from build123d import *

# Parameters (mm, degrees)
PAD_DEPTH = 3
FILLET_R  = 1.25


with BuildPart() as part:
    # Sketch → Pad (new body)
    with BuildSketch(Plane.XY):
        with BuildLine():
            Line((0, 0), (0, 14))
            Line((0, 14), (40, 14))
            Line((40, 14), (40, 6))
            ThreePointArc((40, 6), (42, 4), (44, 6))
            Line((44, 6), (44, 13.953997))
            Line((44, 13.953997), (49, 13.953997))
            Line((49, 13.953997), (49, 6))
            ThreePointArc((42, -1), (46.949747, 1.050253), (49, 6))
            Line((16.769501, -1), (42, -1))
            ThreePointArc((16.769501, -1), (12.734056, -2.671536), (11.06252, -6.706981))
            Line((11.06252, -6.706981), (11.06252, -8))
            Line((5.5, -8), (11.06252, -8))
            Line((5.5, 8), (5.5, -8))
            Line((3, 8), (5.5, 8))
            Line((3, 0), (3, 8))
            Line((0, 0), (3, 0))
        make_face()
    extrude(amount=PAD_DEPTH)

    # Fillet
    fillet_edges = [part.edges().sort_by_distance(p)[0] for p in [
        (20, 14, 3),
        (20, 14, 0),
        (40, 14, 1.5),
        (40, 10, 0),
        (40, 10, 3),
        (42, 4, 0),
        (42, 4, 3),
        (44, 13.953997, 1.5),
        (44, 9.976998, 0),
        (44, 9.976998, 3),
        (49, 13.953997, 1.5),
        (46.5, 13.953997, 0),
        (46.5, 13.953997, 3),
        (49, 9.976998, 0),
        (49, 9.976998, 3),
        (46.949747, 1.050253, 0),
        (46.949747, 1.050253, 3),
        (29.38475, -1, 0),
        (29.38475, -1, 3),
        (12.734056, -2.671536, 0),
        (12.734056, -2.671536, 3),
        (11.06252, -8, 1.5),
        (11.06252, -7.353491, 0),
        (11.06252, -7.353491, 3),
    ]]
    fillet(fillet_edges, radius=FILLET_R)


solid = part.part
The model under review builds one solid part; all positions refer to its coordinate system, in mm. A direction names the side the tool comes from. Give positions to 0.01 mm unless a question says otherwise; leave off trailing zeros. Write each loop counter-clockwise with the first axis right and the second up, starting at its lowest first coordinate (ties: lowest second). Pieces come first, ordered by that corner, then holes.
1. Add section A-A, the plane y = 9. Write out the cut boundary in (x, z).
2. Wall thickness on L1, parallel to X at y = 9, z = 1.3; L2, parallel to X at y = 12, z = 2.5; L3, parallel to Y at x = 35.5, z = 1.5: over which ranges is each line inside the solid? List them lowest first.
3. For P1, Ø6, axis at x = 29.5, y = -3.5, coming from the -Z side; P2, Ø1.5, axis at x = 1.5, z = 1, coming from the -Y side; P3, Ø0.6, axis at x = 46.5, z = 1.5, coming from the +Y side, all flat-tipped, find the tip position at first contact; note any pin that passes through.
4. Tool access review of faces 1 (the cylindrical face through (10.541, -7.219, 2.766)), 2 (the cylindrical face through (39.624, 13.644, 1.504)), 3 (the cylindrical face through (44.356, 9.399, 0.376)): name each direction out of +Z, -Z, +X, -X, +Y, -Y from which nothing blocks a thin tool from reaching the whole face with its end or side.
5. Add section B-B, the plane z = 0.45. Write out the cut boundary in (x, y), plus the area to 3 significant figures.
6. Draft analysis for pull direction Y (two halves, no side actions). For faces 4 (the cylindrical face through (48.62, 13.6, 1.5)), 5 (the flat face through (19, 5, 0)), 6 (the cylindrical face through (29.208, -0.644, 0.376)), state which applies: +Y half, -Y half, draft (parallel to the pull), parting line (faces both ways), or undercut.
Worked answers:
1. outline: (0, 0) - (38.75, 0) arc R1.25 ccw to (40, 1.25) - (40, 1.75) arc R1.25 ccw to (38.75, 3) - (0, 3) - close; (44, 1.25) arc R1.25 ccw to (45.25, 0) - (47.75, 0) arc R1.25 ccw to (49, 1.25) - (49, 1.75) arc R1.25 ccw to (47.75, 3) - (45.25, 3) arc R1.25 ccw to (44, 1.75) - close
2. L1: x = 0 to 40, 44 to 49
2. L2: x = 0 to 39.75, 44.25 to 48.75
2. L3: y = -1 to 14
3. P1: stops at z = 0.25
3. P2: stops at y = 0
3. P3: stops at y = 13.95
4. face 1: +Z, +X, -Y
4. face 2: +Z, -Z, +Y
4. face 3: -Z, +Y
5. outline: (0, 0) - (3, 0) - (3, 8) - (5.5, 8) - (5.5, -8) - (9.81, -8) arc R1.25 ccw to (10.77, -7.55) - (10.77, -6.71) arc R6 cw to (16.77, -0.71) - (42, -0.71) arc R6.71 ccw to (48.71, 6) - (48.71, 12.7) arc R0.96 ccw to (47.75, 13.66) - (45.25, 13.66) arc R0.96 ccw to (44.29, 12.7) - (44.29, 6) arc R2.29 cw to (39.71, 6) - (39.71, 12.75) arc R0.96 ccw to (38.75, 13.71) - (0, 13.71) - close
5. area: 671 mm2
6. face 4: +Y half
6. face 5: draft
6. face 6: -Y half
